Can you work these out from the model? Positions are in its coordinate system, mm. A direction names the side the tool comes from. Coordinates: 2 decimals unless noted, no trailing zeros. Loops run counter-clockwise (first coordinate to the right, second up) from the corner with the lowest first, then second, coordinate; pieces in that order, holes last.
```python
from build123d import *

# Parameters (mm, degrees)
F0_W     = 4.935211
F0_H     = 10.95
F0_W_2   = 5
F0_H_2   = 5
F0_H_3   = 11
F1_DEPTH = 1


with BuildPart() as f1:
    # F0 (on Top) → F1 (new body)
    with BuildSketch(Plane.XY):
        with BuildLine():
            ThreePointArc((41.749027, -33.215299), (44.791117, -31.531696), (46, -28.271721))
            Line((46, -28.271721), (46, -2.5))
            Line((46, -2.5), (43.820465, -2.5))
            ThreePointArc((43.820465, -2.5), (43.515288, -2.452296), (43.239227, -2.313733))
            Line((43.239227, -2.313733), (40.569613, -0.406867))
            ThreePointArc((40.569613, -0.406867), (40.360233, 0), (40.569613, 0.406867))
            Line((40.569613, 0.406867), (43.239227, 2.313733))
            ThreePointArc((43.239227, 2.313733), (43.515288, 2.452296), (43.820465, 2.5))
            Line((43.820465, 2.5), (46, 2.5))
            Line((46, 2.5), (46, 28.271721))
            ThreePointArc((46, 28.271721), (44.791117, 31.531696), (41.749027, 33.215299))
            Line((41.749027, 33.215299), (27, 35.45))
            Line((27, 35.45), (2.75, 35.45))
            Line((2.75, 35.45), (2.75, 32.95))
            Line((2.75, 32.95), (0, 32.95))
            Line((0, 32.95), (-2.75, 32.95))
            Line((-2.75, 32.95), (-2.75, 35.45))
            Line((-2.75, 35.45), (-27.064789, 35.45))
            Line((-27.064789, 35.45), (-41.751913, 33.215906))
            ThreePointArc((-41.751913, 33.215906), (-44.792068, 31.531634), (-46, 28.272766))
            Line((-46, 28.272766), (-46, 2.5))
            Line((-46, 2.5), (-43.820465, 2.5))
            ThreePointArc((-43.820465, 2.5), (-43.515288, 2.452296), (-43.239227, 2.313733))
            Line((-43.239227, 2.313733), (-40.569613, 0.406867))
            ThreePointArc((-40.569613, 0.406867), (-40.360233, 0), (-40.569613, -0.406867))
            Line((-40.569613, -0.406867), (-43.239227, -2.313733))
            ThreePointArc((-43.239227, -2.313733), (-43.515288, -2.452296), (-43.820465, -2.5))
            Line((-43.820465, -2.5), (-46, -2.5))
            Line((-46, -2.5), (-46, -28.272766))
            ThreePointArc((-46, -28.272766), (-44.792068, -31.531634), (-41.751913, -33.215906))
            Line((-41.751913, -33.215906), (-27.064789, -35.45))
            Line((-27.064789, -35.45), (-2.75, -35.45))
            Line((-2.75, -35.45), (-2.75, -32.95))
            Line((-2.75, -32.95), (0, -32.95))
            Line((0, -32.95), (2.75, -32.95))
            Line((2.75, -32.95), (2.75, -35.45))
            Line((2.75, -35.45), (27, -35.45))
            Line((27, -35.45), (41.749027, -33.215299))
        make_face()
        with Locations((-29.532394, -14.975)):
            Rectangle(F0_W, F0_H, mode=Mode.SUBTRACT)
        with Locations((-34.6, -6.9)):
            Rectangle(F0_W_2, F0_H_2, mode=Mode.SUBTRACT)
        with Locations((34.6, 6.85)):
            Rectangle(F0_W_2, F0_H_2, mode=Mode.SUBTRACT)
        with Locations((29.5, 14.95)):
            Rectangle(F0_W_2, F0_H_3, mode=Mode.SUBTRACT)
    extrude(amount=F1_DEPTH)


solid = f1.part
```
Item 1: Suppose I cut it at B-B, the plane x = 35. Please give me the cut outline in (y, z).
Results are:
outline: (-34.24, 0) - (4.35, 0) - (4.35, 1) - (-34.24, 1) - close; (9.35, 0) - (34.24, 0) - (34.24, 1) - (9.35, 1) - close
Item 2: I need wall thicknesses on line 1 along X through (y, z) = (-16, 0.3); line 2 along X through (y, z) = (16, 0.1); line 3 along Y through (x, z) = (2, 0.8). Which ranges of each line are inside material? Lowest first, please.
Results are:
line 1: x = -46 to -32, -27.06 to 46
line 2: x = -46 to 27, 32 to 46
line 3: y = -32.95 to 32.95
Item 3: On a 3-axis mill with a long thin cutter (end or side, diameter ignored), from which of +Z, -Z, +X, -X, +Y, -Y can I reach the whole of each face in a straight line? I mean faces 4 (the face through (-41.89, -1.35, 0.49)), 5 (the face through (44.76, -31.57, 0.49)), 6 (the face through (41.89, 1.35, 0.49)). Say none if no direction works.
Results are:
face 4: +Z, -Z, -X
face 5: +Z, -Z, +X, -Y
face 6: +Z, -Z, +X
Item 4: Suppose I cut it at C-C, the plane z = 0.3. Count the separate pieces of the cut face and the enclosed holes in it, plus the area to 3 significant figures.
Results are:
separate pieces: 1
enclosed holes: 4
area: 6,170 mm2
Item 5: I'm going to push a flat-ended pin straight in: P1, Ø0.5, axis at x = 35.5, z = 0.5, coming from the +Y side. Where does the tip first touch, or does it pass through?
Results are:
P1: stops at y = 34.2
Item 6: We'd pull the mould along Y, two halves only. Please class faces 1 (the face through (-34.511, -34.317, 0.493)), 2 (the face through (-41.92, 1.37, 0.49)), 3 (the face through (-1, 0, 0)): +Y half, -Y half, draft (parallel to the pull), parting line (faces both ways), or undercut.
Results are:
face 1: -Y half
face 2: undercut
face 3: draft
Item 7: Suppose I cut it at A-A, the plane y = 10.5. Please give me the cut outline in (x, z).
Results are:
outline: (-46, 0) - (27, 0) - (27, 1) - (-46, 1) - close; (32, 0) - (46, 0) - (46, 1) - (32, 1) - close
